```python
from build123d import *

# Parameters (mm, degrees)
SKETCH1_R           = 32.5
BOSS_EXTRUDE1_DEPTH = 10
SKETCH4_W           = 40
SKETCH4_H           = 3
BOSS_EXTRUDE3_DEPTH = 40
SKETCH5_R           = 10
CUT_EXTRUDE2_DEPTH  = 40


with BuildPart() as part:
    # Sketch1 → Boss-Extrude1 (new body)
    with BuildSketch(Plane(origin=(0, 0, 0), x_dir=(1, 0, 0), z_dir=(0, 1, 0))):
        with Locations(Location((0, 0, 0), (0, 0, 270))):
            Circle(SKETCH1_R)
    extrude(amount=BOSS_EXTRUDE1_DEPTH)

    # Sketch4 → Boss-Extrude3 (add)
    with BuildSketch(Plane(origin=(0, 10, 0), x_dir=(1, 0, 0), z_dir=(0, 1, 0))):
        Rectangle(SKETCH4_W, SKETCH4_H)
    extrude(amount=BOSS_EXTRUDE3_DEPTH)

    # Sketch5 → Cut-Extrude2 (cut)
    with BuildSketch(Plane.XY.offset(1.5)):
        with Locations((0, 30)):
            Circle(SKETCH5_R)
    extrude(amount=-CUT_EXTRUDE2_DEPTH, mode=Mode.SUBTRACT)


solid = part.part
```
Model file for the job. Use its own axes, mm. A direction names the side the tool comes from. Round coordinates to 2 decimals unless told otherwise and drop trailing zeros. Write each loop counter-clockwise with the first axis right and the second up, starting at its lowest first coordinate (ties: lowest second). Pieces come first, ordered by that corner, then holes. Notation, with made-up numbers: M 61,10 L 74,10 A22 ccw 74,19 Z; hole C 15.25,83.25 d7. An arc over 180 degrees is marked long. Put each result on its own line as item: value.
Item 1: Probe L1, parallel to Y at x = 0, z = -0.6; L2, parallel to Z at x = -17.5, y = 36.5; L3, parallel to Y at x = 5, z = 10.5. List the from-to ranges inside material, lowest first. Write a range as from..to.
Responses:
L1: 0..20, 40..50
L2: -1.5..1.5
L3: 0..10
Item 2: Cut at B-B (x = 0). List the corners of the cut face in (y, z), and give its area (3 significant figures).
Responses:
outline: M 0,-32.5 L 10,-32.5 L 10,-1.5 L 20,-1.5 L 20,1.5 L 10,1.5 L 10,32.5 L 0,32.5 Z; M 40,-1.5 L 50,-1.5 L 50,1.5 L 40,1.5 Z
area: 710 mm²
Item 3: Cut at D-D (y = 21). List the corners of the cut face in (x, z).
Responses:
outline: M -20,-1.5 L -4.36,-1.5 L -4.36,1.5 L -20,1.5 Z; M 4.36,-1.5 L 20,-1.5 L 20,1.5 L 4.36,1.5 Z
Item 4: Mould opens along Y. For faces 5 (the flat face through (-5, 21, 1.5)), 6 (the cylindrical face through (-2.17, 20.24, 0.02)), 7 (the flat face through (0, 50, 0)) say: +Y half, -Y half, draft (parallel to the pull), parting line (faces both ways), or undercut.
Responses:
face 5: draft
face 6: undercut
face 7: +Y half
Item 5: Tool access for faces 1 (the flat face through (-5, 21, -1.5)), 2 (the flat face through (20, 30, 0)), 3 (the flat face through (0, 0, 0)), 4 (the flat face through (-20, 30, 0)): list every direction of +Z, -Z, +X, -X, +Y, -Y with a clear straight run to the whole face (end or side of a thin tool).
Responses:
face 1: -Z, +X, -X, +Y
face 2: +Z, -Z, +X, +Y
face 3: +Z, -Z, +X, -X, -Y
face 4: +Z, -Z, -X, +Y
Item 6: Flat gauge pins, fed straight in: P1, Ø12, axis at x = 19, z = -13, coming from the +Y side; P2, Ø12, axis at x = -5.5, y = 21.5, coming from the +Z side; P3, Ø5, axis at x = -13, y = 7.5, coming from the -Z side. Where does each tip first touch, or does it go through?
Responses:
P1: y = 10
P2: z = 1.5
P3: z = -30.76
Item 7: Cut at C-C (z = 0). List the corners of the cut face in (x, y), and give its area (3 significant figures).
Responses:
outline: M -32.5,0 L 32.5,0 L 32.5,10 L 20,10 L 20,50 L -20,50 L -20,10 L -32.5,10 Z; hole C 0,30 d20
area: 1,940 mm²
Item 8: Cut at A-A (y = 30). List the corners of the cut face in (x, z), and give its area (3 significant figures).
Responses:
outline: M -20,-1.5 L -10,-1.5 L -10,1.5 L -20,1.5 Z; M 10,-1.5 L 20,-1.5 L 20,1.5 L 10,1.5 Z
area: 60.0 mm²
